The figure shows three views and two pictorial views of one solid part (mm, origin at its lowest corner). Answer the questions. A direction names the side the tool comes from. Give positions to 0.01 mm unless a question says otherwise; leave off trailing zeros. Order: outer loops, then holes, each group sorted by start corner. A loop starts at its lowest first (then second) coordinate and runs counter-clockwise, first axis right, second up. Notation, with made-up numbers: (65, 88.5) - (110, 88.5) arc R38 ccw to (110, 126.5) - close; hole circle Ø6 at (-27.75, 74). An arc over 180 degrees is marked (long way). Use a Markdown table: item, result. Add a question column.
1. A cutting plane is placed at C-C on x = 9. Determine the outline of the cut face in (y, z), and give its area (3 significant figures).
2. A cutting plane is placed at D-D on z = 4. Determine the outline of the cut face in (x, y), and give its area (3 significant figures).
3. A cutting plane is placed at A-A on y = 10.25. Determine the outline of the cut face in (x, z).
4. Consider L1, parallel to X at y = 5.3, z = 46.5; L2, parallel to Z at x = 81.5, y = 6.2; L3, parallel to Y at x = 54.5, z = 12. Determine where each line is inside the solid, lowest interval first.
5. Which of the six approach directions +Z, -Z, +X, -X, +Y, -Y give full straight-line access (tool end or side, diameter ignored) to the marked faces 1, 2 and 3?
6. A cutting plane is placed at B-B on z = 44. Determine the outline of the cut face in (x, y).
7. Flat-ended cylindrical pins translate along their axes: P1, Ø1.8, axis at x = 3.5, z = 46.5, coming from the +Y side; P2, Ø3, axis at y = 13, z = 39, coming from the -X side; P3, Ø5.5, axis at y = 9, z = 45, coming from the +X side; P4, Ø25, axis at x = 32.5, z = 23.5, coming from the -Y side. Find the tip coordinate at first contact, or state that the pin passes through.
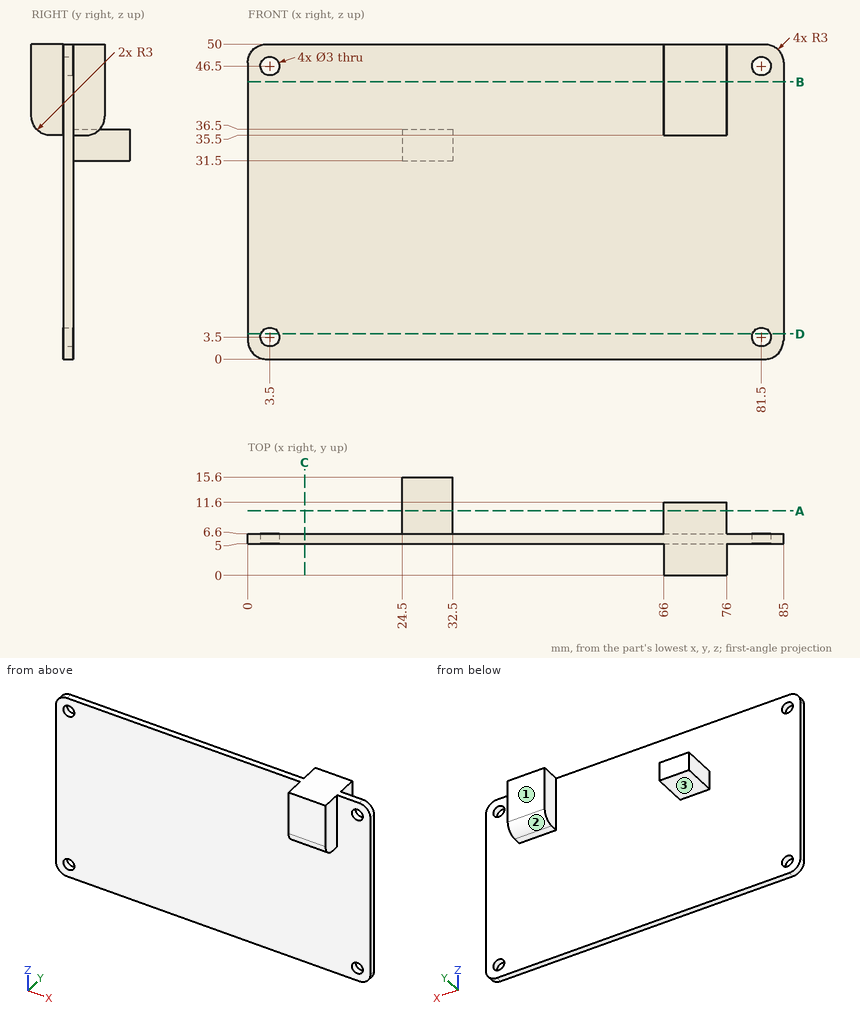
Output values:
| question | item | result |
|---|---|---|
| 1 | outline | (5, 0) - (6.6, 0) - (6.6, 50) - (5, 50) - close |
| 1 | area | 80.0 mm² |
| 2 | outline | (0, 5) - (2.09, 5) - (2.09, 6.6) - (0, 6.6) - close; (4.91, 5) - (80.09, 5) - (80.09, 6.6) - (4.91, 6.6) - close; (82.91, 5) - (85, 5) - (85, 6.6) - (82.91, 6.6) - close |
| 2 | area | 127 mm² |
| 3 | outline | (24.5, 31.5) - (32.5, 31.5) - (32.5, 36.5) - (24.5, 36.5) - close; (66, 35.99) - (76, 35.99) - (76, 50) - (66, 50) - close |
| 4 | L1 | 0 to 2, 5 to 80, 83 to 85 |
| 4 | L2 | 0 to 2, 5 to 45, 48 to 50 |
| 4 | L3 | 5 to 6.6 |
| 5 | face 1 | +Z, -Z, +X, -X, +Y |
| 5 | face 2 | -Z, +X, +Y |
| 5 | face 3 | -Z, +X, -X, +Y |
| 6 | outline | (0, 5) - (66, 5) - (66, 0) - (76, 0) - (76, 5) - (85, 5) - (85, 6.6) - (76, 6.6) - (76, 11.6) - (66, 11.6) - (66, 6.6) - (0, 6.6) - close |
| 7 | P1 | through |
| 7 | P2 | x = 66 |
| 7 | P3 | x = 85 |
| 7 | P4 | y = 5 |
